Could you check a few things on this model? Use its own coordinates, in mm. Give positions to 0.01 mm unless a question says otherwise; leave off trailing zeros. Write each loop counter-clockwise with the first axis right and the second up, starting at its lowest first coordinate (ties: lowest second). Pieces come first, ordered by that corner, then holes. Notation, with made-up numbers: (46.25, -16) -> (54.25, -16) arc R19 ccw to (54.25, 2) -> close; hole circle Ø6 at (32.25, -10). An arc over 180 degrees is marked (long way). One line per question, with ' | ' between items.
from build123d import *

# Parameters (mm, degrees)
SKETCH1_R           = 1.778
BOSS_EXTRUDE1_DEPTH = 101.6
SKETCH2_R           = 2.794
SKETCH2_W           = 25.4
SKETCH2_H           = 6.35
CUT_EXTRUDE1_DEPTH  = 914.4
LPATTERN1_COUNT     = 3
LPATTERN1_PITCH     = 50.8
LPATTERN2_COUNT     = 3
LPATTERN2_PITCH     = 50.8


with BuildPart() as part:
    # Sketch1 → Boss-Extrude1 (new body, symmetric)
    with BuildSketch(Plane(origin=(0, 0, 0), x_dir=(0, 0, -1), z_dir=(1, 0, 0))):
        with BuildLine():
            Line((0, -2.794), (25.4, -2.794))
            Line((25.4, -2.794), (25.4, -1.778))
            Line((25.4, -1.778), (2.155261469, -1.778))
            ThreePointArc((2.155261469, -1.778), (-1.191365603, 2.52726809), (0, -2.794))
        make_face()
        Circle(SKETCH1_R, mode=Mode.SUBTRACT)
    extrude(amount=BOSS_EXTRUDE1_DEPTH, both=True)

    # Sketch2 → Cut-Extrude1 (cut, symmetric)
    with BuildSketch(Plane(origin=(0, -1.778, 0), x_dir=(1, 0, 0), z_dir=(0, 1, 0))):
        with Locations((-25.4, 14.224)):
            Circle(SKETCH2_R)
        with Locations((-12.7, 0.381)):
            Rectangle(SKETCH2_W, SKETCH2_H)
    cut_extrude1 = extrude(amount=CUT_EXTRUDE1_DEPTH, both=True, mode=Mode.SUBTRACT)

    # LPattern1: Cut-Extrude1 ×3
    with Locations(*[(-i * LPATTERN1_PITCH, 0, 0) for i in range(1, LPATTERN1_COUNT)]):
        add(cut_extrude1, mode=Mode.SUBTRACT)

    # LPattern2: Cut-Extrude1 ×3
    with Locations(*[(i * LPATTERN2_PITCH, 0, 0) for i in range(1, LPATTERN2_COUNT)]):
        add(cut_extrude1, mode=Mode.SUBTRACT)


solid = part.part
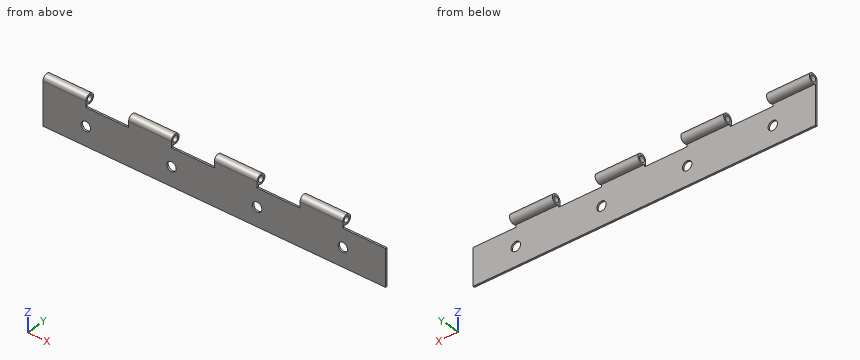
Q1. If I drill on line 1 along X through (y, z) = (1.65, -1.25); line 2 along Z through (x, y) = (5.5, 0); line 3 along Y through (x, z) = (85, -14), over which ranges is the centre line in solid material (lowest first)?
Answer below:
line 1: x = -101.6 to -76.2, -50.8 to -25.4, 0 to 25.4, 50.8 to 76.2 | line 2: z = -2.79 to -1.78, 1.78 to 2.79 | line 3: y = -2.79 to -1.78
Q2. Will these pins go through, and if not, where does the flat tip stop? pin 1 (1.7 mm diameter, centred on y = 0.5, z = -1, fed in from +X); pin 2 (7 mm diameter, centred on x = -51, z = -18.5, fed in from +Y); pin 3 (0.5 mm diameter, centred on x = 83.5, y = -2.5, fed in from +Z).
Answer below:
pin 1: stops at x = 76.2 | pin 2: stops at y = -1.78 | pin 3: stops at z = -3.56
Q3. Imagine slicing it at C-C on x = -14. Please give me the cut outline in (y, z).
Answer below:
outline: (-2.79, -25.4) -> (-1.78, -25.4) -> (-1.78, -3.56) -> (-2.79, -3.56) -> close
Q4. Imagine slicing it at A-A on x = -48. Please give me the cut outline in (y, z), and give its area (3 significant figures).
Answer below:
outline: (-2.79, -25.4) -> (-1.78, -25.4) -> (-1.78, -2.16) arc R2.79 ccw (long way) to (-2.79, 0) -> close; hole circle Ø3.56 at (0, 0) | area: 38.9 mm^2
Q5. Imagine slicing it at B-B on z = -20.75. Please give me the cut outline in (x, y).
Answer below:
outline: (-101.6, -2.79) -> (101.6, -2.79) -> (101.6, -1.78) -> (-101.6, -1.78) -> close
